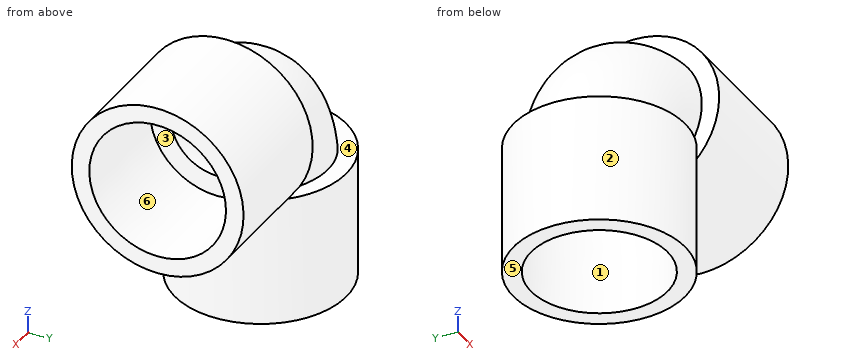
Autodesk Inventor part; units mm, degrees
ref_plane "YZ Plane" through (0, 0, 0) normal (1, 0, 0) x (0, 1, 0)
ref_plane "XZ Plane" through (0, 0, 0) normal (0, 1, 0) x (-1, 0, 0)
ref_plane "XY Plane" through (0, 0, 0) normal (0, 0, 1) x (1, 0, 0)
sketch "Sketch1" plane through (0, 0, 0) normal (0, 1, 0) x (-1, 0, 0)
  line L0 (0, 0) -> (0, 17.4752)
  arc A0 (0, 17.4752) -> (-12.7, 30.1752) centre (-12.7, 17.4752) ccw
  line L1 (-12.7, 30.1752) -> (-30.1752, 30.1752)
  line L2 (-12.7, 30.1752) -> (0, 30.1752) construction
  line L3 (0, 30.1752) -> (0, 17.4752) construction
  dimension "d0" = 30.1752
  dimension "d1" = 30.1752
  dimension "d2" = 17.4752
sketch "Sketch2" plane through (0, 0, 0) normal (0, 0, 1) x (1, 0, 0)
  circle A0 centre (0, 0) radius 10.795
  circle A1 centre (0, 0) radius 7.3406
  dimension "d3" = 14.6812
  dimension "d4" = 21.59
sweep "Sweep1" add profiles "Sketch2" path "Sketch1"
sketch "Sketch3" plane through (0, 0, 0) normal (0, 0, -1) x (-1, 0, 0)
  circle A0 centre (0, 0) radius 13.5382
  circle A1 centre (0, 0) radius 10.795
  circle A2 centre (0, 0) radius 9.0678
  dimension "d6" = 27.0764
  dimension "d9" = 18.1356
extrude "Extrusion1" add sketch "Sketch3" against normal blind 20.2438 contours A0 | A1
sketch "Sketch4" plane through (30.1752, 0, 30.1752) normal (1, 0, 0) x (0, 0, -1)
  circle A0 centre (0, 0) radius 7.3406
  circle A1 centre (0, 0) radius 9.0678
  circle A2 centre (0, 0) radius 13.5382
  dimension "d10" = 27.0764
  dimension "d11" = 18.1356
extrude "Extrusion2" add sketch "Sketch4" against normal blind 20.2438 contours A2
sketch "Sketch5" plane through (0, 0, 0) normal (0, 0, -1) x (-1, 0, 0)
  circle A0 centre (0, 0) radius 7.3406
  circle A1 centre (0, 0) radius 10.7696
  dimension "d14" = 21.5392
sketch "Sketch5 outline for Extrusion3" plane through (0, 0, 0) normal (0, 0, -1) x (-1, 0, 0)
  circle A0 centre (0, 0) radius 10.7696
extrude "Extrusion3" cut sketch "Sketch5 outline for Extrusion3" against normal blind 17.4752 draft -0.49966
sketch "Sketch6" plane through (30.1752, 0, 30.1752) normal (1, 0, 0) x (0, 0, -1)
  circle A0 centre (0, 0) radius 7.3406
  circle A1 centre (0, 0) radius 10.7696
  dimension "d17" = 21.5392
sketch "Sketch6 outline for Extrusion4" plane through (30.1752, 0, 30.1752) normal (1, 0, 0) x (0, 0, -1)
  circle A0 centre (0, 0) radius 10.7696
extrude "Extrusion4" cut sketch "Sketch6 outline for Extrusion4" against normal blind 17.4752 draft -0.49966
equation "\"d0\" = G + C1"
equation "\"d1\" = G + C1"
equation "\"d2\" = C1"
equation "\"d3\" = D"
equation "\"d4\" = D + 2 * F1"
equation "\"d6\" = A + 2 * E1"
equation "\"d9\" = D + F1"
equation "\"d7\" = C1 + E1"
equation "\"d10\" = A + 2 * E1"
equation "\"d11\" = D + F1"
equation "\"d12\" = C1 + E1"
equation "\"d14\" = A"
equation "\"d15\" = C1"
equation "\"d17\" = A"
equation "\"d18\" = C1"
equation "\"A\" = 21.5392"
equation "\"C1\" = 17.4752"
equation "\"F1\" = 3.4544"
equation "\"D\" = 14.6812"
equation "\"G\" = 12.7"
equation "\"E1\" = 2.7686"
equation "\"B\" = 21.2344"
equation "\"Size_Designation\" = 0.5"
properties part number "ASTM D 2466 90 Deg Elbow Socket-Type - Schedule 40 1/2" material "PVC-Piping"
Check sheet for the modelled part. Datum: model origin and axes. Units: mm. Face numbers are marked on the shaded views. A direction names the side the tool comes from. Coordinates: 2 decimals unless noted, no trailing zeros. Write each loop counter-clockwise with the first axis right and the second up, starting at its lowest first coordinate (ties: lowest second). Pieces come first, ordered by that corner, then holes. Notation, with made-up numbers: M -1.75,59.5 L 12.25,59.5 A21 cw 12.25,97.5 Z; hole C 31,89.25 d1. An arc over 180 degrees is marked long. Write item = value, one per line. Start each with the question number.
1. Go/stop test with flat-tipped pins: pin 1 (10 mm diameter, centred on y = -3, z = 12, fed in from +X); pin 2 (5 mm diameter, centred on x = 24.5, z = 35.5, fed in from -Y); pin 3 (12 mm diameter, centred on x = -1, y = 1.5, fed in from -Z); pin 4 (6 mm diameter, centred on x = -5, z = 31.5, fed in from -Y). Record where each tip stops, or that it passes through.
2. Sectioned sample at B-B (x = 19). Record the cut outline in (y, z), then the cut area to 3 significant figures.
3. Mould release check, pull along X, two halves, no side actions. Record for the marked faces 1, 2 and 3: pulls with the +X half, pulls with the -X half, needs draft (parallel to the pull), parting line crosses it, or undercut.
4. Tool access check on the marked faces 4, 5 and 6. Record the directions out of +Z, -Z, +X, -X, +Y, -Y that give a thin tool (end or side, any length) a straight path to the whole face; none if there is none.
5. Thickness scan on probe 1 along Y at (x, z) = (13.5, 30); probe 2 along X at (y, z) = (-4, 11); probe 3 along X at (y, z) = (2.25, 12.5). Record the ranges inside material, lowest first.
6. Sectioned sample at A-A (z = 3). Record the cut outline in (x, y).
The answers:
q1.pin_1 = 30.18
q1.pin_2 = -13.24
q1.pin_3 = 17.48
q1.pin_4 = -8.32
q2.outline = C 0,30.18 d27.08; hole C 0,30.18 d21.34
q2.area = 218 mm²
q3.face_1 = undercut
q3.face_2 = parting line crosses it
q3.face_3 = pulls with the +X half
q4.face_4 = none
q4.face_5 = -Z, +X, -X, +Y, -Y
q4.face_6 = +X
q5.probe_1 = -13.54 to -10.62, 10.62 to 13.54
q5.probe_2 = -12.93 to -9.9, 9.9 to 12.93
q5.probe_3 = -13.35 to -10.42, 10.42 to 13.35
q6.outline = C 0,0 d27.08; hole C 0,0 d21.49
